The listing builds one solid part. Answer for the finished solid, in the listing's coordinates (mm). A direction names the side the tool comes from. Give positions to 0.01 mm unless a question says otherwise; leave off trailing zeros. Order: outer loops, then holes, each group sorted by start corner. A loop starts at its lowest first (then second) coordinate and runs counter-clockwise, first axis right, second up. Notation, with made-up numbers: (12, 85.5) -> (68, 85.5) arc R24 cw to (68, 101.5) -> close; hole circle Ø6 at (12.5, -7). An arc over 180 degrees is marked (long way). One line per question, with ' | ' between items. Start each with the question number.
```python
from build123d import *

# Parameters (mm, degrees)
SKETCH1_R           = 4.4
SKETCH1_R_2         = 2.55
SKETCH1_W           = 1.8
SKETCH1_H           = 0.2
BOSS_EXTRUDE1_DEPTH = 4


with BuildPart() as part:
    # Sketch1 → Boss-Extrude1 (new, symmetric)
    # profile 1 of 3: a face of its own
    with BuildSketch(Plane(origin=(0, 0, 0), x_dir=(1, 0, 0), z_dir=(0, 1, 0))):
        with Locations(Location((0, 0, 0), (0, 0, 270))):
            Circle(SKETCH1_R)
        Circle(SKETCH1_R_2, mode=Mode.SUBTRACT)
    # profile 2 of 3: a face of its own
    with BuildSketch(Plane(origin=(0, 0, 0), x_dir=(1, 0, 0), z_dir=(0, 1, 0))):
        with Locations((0, 2.285896058)):
            Rectangle(SKETCH1_W, SKETCH1_H)
    # profile 3 of 3: a face of its own
    with BuildSketch(Plane(origin=(0, 0, 0), x_dir=(1, 0, 0), z_dir=(0, 1, 0))):
        with BuildLine():
            ThreePointArc((0.9, 2.385896058), (0, 2.55), (-0.9, 2.385896058))
            Line((-0.9, 2.385896058), (0.9, 2.385896058))
        make_face()
    extrude(amount=BOSS_EXTRUDE1_DEPTH, both=True)


solid = part.part
```
(1) Given P1, Ø3, axis at x = -2.5, y = -2, coming from the +Z side; P2, Ø1, axis at x = 1.5, y = 1, coming from the -Z side; P3, Ø1, axis at y = -1, z = -2.5, coming from the -X side, each flat-ended and moving along its own axis, determine where each tip first touches the part or whether it passes through.
(2) Consider line 1 (X direction, y = 0.5, z = 0); line 2 (Z direction, x = 0.25, y = 3); line 3 (Z direction, x = 2.25, y = 1). Determine where each line is inside the solid, lowest interval first.
(3) Determine the mould class of faces 3 (the face through (-0.1, 0.06, 2.55)), 4 (the face through (4.363, 0.056, -0.573)), 5 (the face through (-2, 4, 2)) for opening direction X: pulls with the +X half, pulls with the -X half, needs draft (parallel to the pull), parting line crosses it, or undercut.
(4) For faces 1 (the face through (2, -4, 2)), 2 (the face through (0, 0, -2.186)), determine the directions among +Z, -Z, +X, -X, +Y, -Y from which every point of the face is accessible in a straight line to the end or side of a thin tool.
(5) The part is cut by section B-B on z = 0. Determine the outline of the cut face in (x, y).
(6) The part is cut by section C-C on y = 2. Determine the outline of the cut face in (x, z).
(7) The part is cut by section A-A on x = 0. Determine the outline of the cut face in (y, z), plus the area to 3 significant figures.
(8) The part is cut by section D-D on z = 3. Determine the outline of the cut face in (x, y).
Result sheet:
1) P1: stops at z = 4.28 | P2: stops at z = -4.28 | P3: stops at x = -3.92
2) line 1: x = -4.4 to -2.55, 2.55 to 4.4 | line 2: z = -4.39 to -2.19, 2.54 to 4.39 | line 3: z = -3.78 to -1.2, 1.2 to 3.78
3) face 3: undercut | face 4: parting line crosses it | face 5: needs draft
4) face 1: +Z, -Z, +X, -X, -Y | face 2: +Y, -Y
5) outline: (-4.4, -4) -> (-2.55, -4) -> (-2.55, 4) -> (-4.4, 4) -> close; (2.55, -4) -> (4.4, -4) -> (4.4, 4) -> (2.55, 4) -> close
6) outline: circle Ø8.8 at (0, 0); hole (-0.9, -2.39) -> (-0.9, -2.19) -> (0.9, -2.19) -> (0.9, -2.39) arc R2.55 ccw (long way) to start
7) outline: (-4, -4.4) -> (4, -4.4) -> (4, -2.19) -> (-4, -2.19) -> close; (-4, 2.55) -> (4, 2.55) -> (4, 4.4) -> (-4, 4.4) -> close | area: 32.5 mm^2
8) outline: (-3.22, -4) -> (3.22, -4) -> (3.22, 4) -> (-3.22, 4) -> close
